Verification items for the finished model (mm, model axes). A direction names the side the tool comes from. Round coordinates to 2 decimals unless told otherwise and drop trailing zeros. Loops run counter-clockwise (first coordinate to the right, second up) from the corner with the lowest first, then second, coordinate; pieces in that order, holes last. Notation, with made-up numbers: M -19,-11 L 8,-11 A36 ccw 8,25 Z; hole C 83.5,73 d6. An arc over 180 degrees is marked long. Answer as CSV lines item,"result".
```python
from build123d import *

# Parameters (mm, degrees)
SKETCH1_R           = 2.5
BOSS_EXTRUDE1_DEPTH = 10
SKETCH2_R           = 2.45
BOSS_EXTRUDE2_DEPTH = 20
BOSS_EXTRUDE3_START = -10
SKETCH3_R           = 2.5
BOSS_EXTRUDE3_DEPTH = 10


with BuildPart() as part:
    # Sketch1 → Boss-Extrude1 (new body)
    with BuildSketch(Plane(origin=(0, 0, 0), x_dir=(1, 0, 0), z_dir=(0, 1, 0))):
        Polygon((0, 15), (0, 0), (15, 0), (15, 5), (5, 5), (5, 15), align=None)
        with Locations(Location((2.879948547, 3.000793191, 0), (0, 0, 270))):
            Circle(SKETCH1_R, mode=Mode.SUBTRACT)
    extrude(amount=BOSS_EXTRUDE1_DEPTH)



with BuildPart() as body_2:
    # Sketch2 → Boss-Extrude2 (new body)
    with BuildSketch(Plane(origin=(0, 10, 0), x_dir=(1, 0, 0), z_dir=(0, 1, 0))):
        with Locations(Location((2.879948547, 3.000793191, 0), (0, 0, 270))):
            Circle(SKETCH2_R)
    extrude(amount=-BOSS_EXTRUDE2_DEPTH)


with BuildPart() as part_1:
    add(part.part)

    add(body_2.part)  # Boss-Extrude3 merges body 2
    # Sketch3 → Boss-Extrude3 (add)
    with BuildSketch(Plane(origin=(0, 10, 0), x_dir=(1, 0, 0), z_dir=(0, 1, 0)).offset(BOSS_EXTRUDE3_START)):
        with Locations((2.879948547, 3.000793191)):
            Circle(SKETCH3_R)
    extrude(amount=BOSS_EXTRUDE3_DEPTH)


solid = part_1.part
```
1) Section check D-D (z = -2.5). Record the cut outline in (x, y).
Here are the results:
outline,"M 0,0 L 0.48,0 L 0.48,-10 L 5.28,-10 L 5.28,0 L 15,0 L 15,10 L 0,10 Z"
2) Set-up check for faces 1 (the flat face through (0, 5, -8)), 2 (the cylindrical face through (3.616, -4.93, -0.664)), 3 (the flat face through (5, 5, -10)): record each of +Z, -Z, +X, -X, +Y, -Y from which the full face is reachable in a straight line by a thin tool's end or side.
Here are the results:
face 1,"+Z, -Z, -X, +Y, -Y"
face 2,"-Y"
face 3,"-Z, +X, +Y, -Y"
3) Go/stop test with flat-tipped pins: pin 1 (1.5 mm diameter, centred on y = -7.5, z = -6, fed in from -X); pin 2 (5 mm diameter, centred on x = 8, y = 1, fed in from +Z); pin 3 (6 mm diameter, centred on x = 4, y = -7.5, fed in from -Z); pin 4 (2 mm diameter, centred on y = 1, z = -12, fed in from +X). Record where each tip stops, or that it passes through.
Here are the results:
pin 1,"stops at x = 1.91"
pin 2,"stops at z = 0"
pin 3,"stops at z = -5.45"
pin 4,"stops at x = 5"
4) Section check B-B (z = -13). Record the cut outline in (x, y).
Here are the results:
outline,"M 0,0 L 5,0 L 5,10 L 0,10 Z"
5) Material ranges on probe 1 along Y at (x, z) = (1.5, -7); probe 2 along Z at (x, y) = (5.5, 1.25); probe 3 along X at (y, z) = (2.75, -7.25), recorded low to high.
Here are the results:
probe 1,"y = 0 to 10"
probe 2,"z = -5 to 0"
probe 3,"x = 0 to 5"
6) Section check A-A (y = 0.5). Record the cut outline in (x, z).
Here are the results:
outline,"M 0,-15 L 5,-15 L 5,-5 L 15,-5 L 15,0 L 0,0 Z"
7) Section check C-C (x = 4.5). Record the cut outline in (y, z), plus the area to 3 significant figures.
Here are the results:
outline,"M -10,-4.84 L 0,-4.84 L 0,-15 L 10,-15 L 10,0 L 0,0 L 0,-1.16 L -10,-1.16 Z"
area,"187 mm^2"
